Check sheet for the modelled part. Datum: model origin and axes. Units: mm. Give positions to 0.01 mm unless a question says otherwise; leave off trailing zeros. Write each loop counter-clockwise with the first axis right and the second up, starting at its lowest first coordinate (ties: lowest second). Pieces come first, ordered by that corner, then holes.
from build123d import *

# Parameters (mm, degrees)
SKETCH003_R     = 1.65
PAD002_DEPTH    = 7
SKETCH004_R     = 2.15
POCKET003_DEPTH = 8
FILLET001_R     = 1.5
CHAMFER001_SIZE = 0.3


with BuildPart() as part:
    # Sketch003 → Pad002 (new body)
    with BuildSketch(Plane.XZ):
        with BuildLine():
            ThreePointArc((0, 4.65), (-4.65, 0), (0, -4.65))
            Line((18.300003, -4.65), (0, -4.65))
            ThreePointArc((18.300003, -4.65), (22.95, 2e-06), (18.3, 4.65))
            Line((0, 4.65), (18.3, 4.65))
        make_face()
        Circle(SKETCH003_R, mode=Mode.SUBTRACT)
        with Locations((18.3, 0)):
            Circle(SKETCH003_R, mode=Mode.SUBTRACT)
    extrude(amount=PAD002_DEPTH)

    # Sketch004 (on Face8 of Pad002) → Pocket003 (cut)
    with BuildSketch(Plane.XZ.offset(7)):
        with Locations((9.15, 0)):
            Circle(SKETCH004_R)
    extrude(amount=-POCKET003_DEPTH, mode=Mode.SUBTRACT)

    # Fillet001
    fillet001_edges = [part.edges().sort_by_distance(p)[0] for p in [
        (-4.65, -7, 0),
        (-4.65, 0, 0),
    ]]
    fillet(fillet001_edges, radius=FILLET001_R)

    # Chamfer001
    chamfer001_edges = [part.edges().sort_by_distance(p)[0] for p in [
        (-1.65, -7, 0),
        (16.65, -7, 0),
        (7, 0, 0),
        (-1.65, 0, 0),
        (16.65, 0, 0),
    ]]
    chamfer(chamfer001_edges, length=CHAMFER001_SIZE)


with BuildPart() as part_1:
    # Body001 placement: moved
    add(part.part.moved(Location((0, -66.5, 0))))


solid = part_1.part
1) Scan lines: L1, parallel to Z at x = 9.15, y = -71.25; L2, parallel to Z at x = 0, y = -71.5; L3, parallel to X at y = -72, z = -0.5. Record each from-to range of solid material in increasing order.
2) Draft check along X on faces 1 (the flat face through (6, -66.5, 0)), 2 (the cylindrical face through (7.444, -70.197, -1.308)), 3 (the cylindrical face through (-4.65, -69.97, 0.1)). Enter one of: +X half, -X half, draft (parallel to the pull), parting line (faces both ways), or undercut.
3) Sectioned sample at C-C on x = 4. Record the boundary of the cut face in (y, z), then the cut area to 3 significant figures.
4) Sectioned sample at A-A on y = -71.25. Record the boundary of the cut face in (x, z).
5) Gauge pin test, flat ends, axial feed: pin 1 (1 mm diameter, centred on y = -69, z = -1, fed in from -X); pin 2 (4 mm diameter, centred on x = 18.3, z = 0, fed in from +Y). Record the tip position at first contact, or that the pin passes through.
6) Sectioned sample at D-D on z = -1. Give the number of separate pieces and of enclosed holes in the cut face, then the cut area to 3 significant figures.
7) Sectioned sample at B-B on x = 9.15. Record the boundary of the cut face in (y, z), then the cut area to 3 significant figures.
Answers below:
1. L1: z = -4.65 to -2.15, 2.15 to 4.65
1. L2: z = -4.65 to -1.65, 1.65 to 4.65
1. L3: x = -4.62 to -1.57, 1.57 to 7.06, 11.24 to 16.73, 19.87 to 22.92
2. face 1: draft
2. face 2: undercut
2. face 3: -X half
3. outline: (-73.5, -3.15) arc R1.5 ccw to (-72, -4.65) - (-68, -4.65) arc R1.5 ccw to (-66.5, -3.15) - (-66.5, 3.15) arc R1.5 ccw to (-68, 4.65) - (-72, 4.65) arc R1.5 ccw to (-73.5, 3.15) - close
3. area: 63.2 mm2
4. outline: (0, -4.65) - (18.3, -4.65) arc R4.65 ccw to (18.3, 4.65) - (0, 4.65) arc R4.65 ccw to start; hole circle Ø3.3 at (0, 0); hole circle Ø4.3 at (9.15, 0); hole circle Ø3.3 at (18.3, 0)
5. pin 1: stops at x = -4.62
5. pin 2: stops at y = -66.5
6. separate pieces: 4
6. enclosed holes: 0
6. area: 126 mm2
7. outline: (-73.5, -3.15) arc R1.5 ccw to (-72, -4.65) - (-68, -4.65) arc R1.5 ccw to (-66.5, -3.15) - (-66.5, -2.45) - (-66.8, -2.15) - (-73.5, -2.15) - close; (-73.5, 2.15) - (-66.8, 2.15) - (-66.5, 2.45) - (-66.5, 3.15) arc R1.5 ccw to (-68, 4.65) - (-72, 4.65) arc R1.5 ccw to (-73.5, 3.15) - close
7. area: 33.0 mm2
